Geometry: final body of the model. Coordinates: model frame, mm. Face numbers are marked on the shaded views. A direction names the side the tool comes from. Give positions to 0.01 mm unless a question says otherwise; leave off trailing zeros. Loops run counter-clockwise (first coordinate to the right, second up) from the corner with the lowest first, then second, coordinate; pieces in that order, holes last. Notation, with made-up numbers: (-22, 11) -> (23, 11) arc R10 ccw to (23, 26) -> close; hole circle Ø7 at (-2, -38.5). An arc over 180 degrees is marked (long way). Answer in a Markdown table with one row per item. Add a question column.
1) First-contact query: P1, Ø4, axis at x = 0, z = 0, coming from the -Y side (1 decimal); P2, Ø1, axis at x = -2.5, z = -2.5, coming from the +Y side. Flat tips, straight axial feed; report the tip coordinate or a pass-through.
2) Section query A-A (x = 0). Return the cut outline in (y, z) (3 decimals).
3) Line query: line 1 (X direction, y = 4.5, z = 0) (3 decimals); line 2 (Y direction, x = 6.25, z = -3); line 3 (Y direction, x = -0.5, z = -5). Output: solid intervals per line, ascending. Write a range as from..to.
4) Section query B-B (z = 0). Return the cut outline in (x, y) (3 decimals), plus the area to 3 significant figures.
5) Section query D-D (y = 2). Return the cut outline in (x, z).
6) Section query C-C (y = 5.5). Return the cut outline in (x, z) (3 decimals), plus the area to 3 significant figures.
7) Draft query along Z for the marked faces 1, 2 and 3. Return one class per face: +Z half, -Z half, draft (parallel to the pull), parting line (faces both ways), or undercut.
8) Access query for the marked faces 4 and 5. Directions: +Z, -Z, +X, -X, +Y, -Y. A direction counts if a zero-diameter tool reaches every point of the face in a straight line with its end or side. Return the directions, or none.
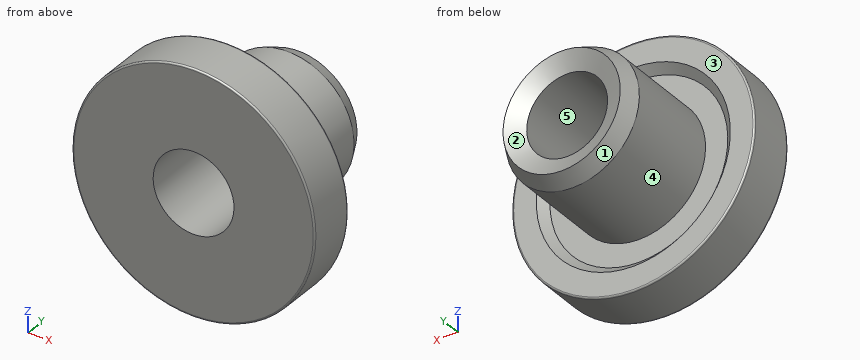
```python
from build123d import *

# Parameters (mm, degrees)
HEADFILLET_R = 0.1


with BuildPart() as part:
    # ProfileS → Profile (revolve)
    with BuildSketch(Plane.XY, mode=Mode.PRIVATE) as profile_sk:
        Polygon((2.5, 0), (7.5, 0), (7.5, 3), (6, 3), (5.5, 2.5), (4.125, 2.5), (4.125, 8.5), (3.625, 9.5), (2.5, 9), align=None)
    revolve(profile_sk.sketch.rotate(Axis((0, 0, 0), (0, 1, 0)), 90), axis=Axis((0, 0, 0), (0, 1, 0)))

    # HeadFillet
    headfillet_edges = [part.edges().sort_by_distance(p)[0] for p in [
        (0, 3, 7.5),
        (0, 0, 7.5),
    ]]
    fillet(headfillet_edges, radius=HEADFILLET_R)


solid = part.part
```
Evaluation:
| question | item | result |
|---|---|---|
| 1 | P1 | through |
| 1 | P2 | y = 9.5 |
| 2 | outline | (0, -7.4) arc R0.1 ccw to (0.1, -7.5) -> (2.9, -7.5) arc R0.1 ccw to (3, -7.4) -> (3, -6) -> (2.5, -5.5) -> (2.5, -4.125) -> (8.5, -4.125) -> (9.5, -3.625) -> (9, -2.5) -> (0, -2.5) -> close; (0, 2.5) -> (9, 2.5) -> (9.5, 3.625) -> (8.5, 4.125) -> (2.5, 4.125) -> (2.5, 5.5) -> (3, 6) -> (3, 7.4) arc R0.1 ccw to (2.9, 7.5) -> (0.1, 7.5) arc R0.1 ccw to (0, 7.4) -> close |
| 3 | line 1 | -4.125..-2.5, 2.5..4.125 |
| 3 | line 2 | 0..3 |
| 3 | line 3 | 0..2.5 |
| 4 | outline | (-7.5, 0.1) arc R0.1 ccw to (-7.4, 0) -> (-2.5, 0) -> (-2.5, 9) -> (-3.625, 9.5) -> (-4.125, 8.5) -> (-4.125, 2.5) -> (-5.5, 2.5) -> (-6, 3) -> (-7.4, 3) arc R0.1 ccw to (-7.5, 2.9) -> close; (2.5, 0) -> (7.4, 0) arc R0.1 ccw to (7.5, 0.1) -> (7.5, 2.9) arc R0.1 ccw to (7.4, 3) -> (6, 3) -> (5.5, 2.5) -> (4.125, 2.5) -> (4.125, 8.5) -> (3.625, 9.5) -> (2.5, 9) -> close |
| 4 | area | 48.4 mm² |
| 5 | outline | circle Ø15 at (0, 0); hole circle Ø5 at (0, 0) |
| 6 | outline | circle Ø8.25 at (0, 0); hole circle Ø5 at (0, 0) |
| 6 | area | 33.8 mm² |
| 7 | face 1 | parting line |
| 7 | face 2 | undercut |
| 7 | face 3 | draft |
| 8 | face 4 | +Y |
| 8 | face 5 | +Y, -Y |
